Geometry: see drawing. Coordinates: mm, zero at the bounding-box minimum. Coordinates: 2 decimals unless noted, no trailing zeros. Order: outer loops, then holes, each group sorted by start corner. A loop starts at its lowest first (then second) coordinate and runs counter-clockwise, first axis right, second up.
Item 1: Ray query, line 1 (Y direction, x = 14, z = 2.15); line 2 (Y direction, x = 14, z = 6); line 3 (X direction, y = 19.25, z = 1). Return the intervals inside material, ascending.
Item 2: Section C-C on x = 25. Return the cut outline in (y, z) (1 decimal).
Item 3: Section A-A on x = 14. Return the cut outline in (y, z).
Item 4: Section D-D on z = 14.25. Return the cut outline in (x, y).
Item 5: Section B-B on y = 14. Return the cut outline in (x, z).
Item 6: Mould query, pull axis X, two halves, no side actions, for the marked faces 1, 2 and 3. Classes: released by +X, released by -X, zero draft, split by the parting line, or undercut.
Item 7: Contact query for flat-ended pins moving along their axis: P1, Ø3.5, axis at x = 4.04, y = 19.75, coming from the -Z side; P2, Ø5, axis at x = 4.04, y = 8.25, coming from the +Z side; P3, Ø3, axis at x = 15.5, z = 10.5, coming from the +Y side; P4, Ø3, axis at x = 20.5, z = 12, coming from the -Y side. Output: stop coordinate, or through.
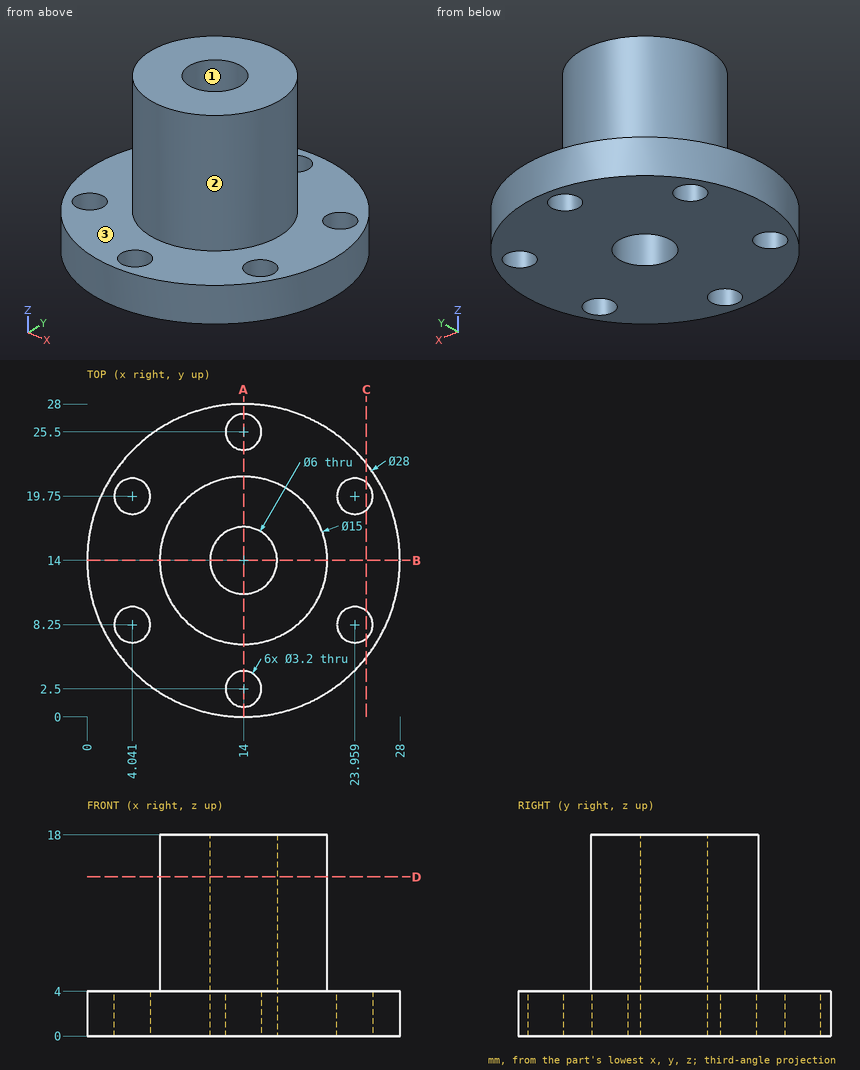
Answer list:
1. line 1: y = 0 to 0.9, 4.1 to 11, 17 to 23.9, 27.1 to 28
1. line 2: y = 6.5 to 11, 17 to 21.5
1. line 3: x = 1.02 to 2.52, 5.56 to 22.44, 25.48 to 26.98
2. outline: (5.3, 0) - (7, 0) - (7, 4) - (5.3, 4) - close; (9.5, 0) - (18.5, 0) - (18.5, 4) - (9.5, 4) - close; (21, 0) - (22.7, 0) - (22.7, 4) - (21, 4) - close
3. outline: (0, 0) - (0.9, 0) - (0.9, 4) - (0, 4) - close; (4.1, 0) - (11, 0) - (11, 18) - (6.5, 18) - (6.5, 4) - (4.1, 4) - close; (17, 0) - (23.9, 0) - (23.9, 4) - (21.5, 4) - (21.5, 18) - (17, 18) - close; (27.1, 0) - (28, 0) - (28, 4) - (27.1, 4) - close
4. outline: circle Ø15 at (14, 14); hole circle Ø6 at (14, 14)
5. outline: (0, 0) - (11, 0) - (11, 18) - (6.5, 18) - (6.5, 4) - (0, 4) - close; (17, 0) - (28, 0) - (28, 4) - (21.5, 4) - (21.5, 18) - (17, 18) - close
6. face 1: undercut
6. face 2: split by the parting line
6. face 3: zero draft
7. P1: stops at z = 0
7. P2: stops at z = 4
7. P3: stops at y = 21.5
7. P4: stops at y = 8.41
